Work out the finished part from the listing and answer in its coordinate system (mm). A direction names the side the tool comes from. Coordinates: 2 decimals unless noted, no trailing zeros. Loops run counter-clockwise (first coordinate to the right, second up) from the corner with the lowest first, then second, coordinate; pieces in that order, holes last. Notation, with made-up numbers: (85, 66) -> (136, 66) arc R23 ccw to (136, 86) -> close; hole circle Ø1 at (-11, 58). An arc over 180 degrees is marked (long way). Use a Markdown table: item, result.
from build123d import *

# Parameters (mm, degrees)
PAD003_DEPTH    = 975
SKETCH013_W     = 310
SKETCH013_H     = 1100
SKETCH013_W_2   = 5
SKETCH013_H_2   = 42.9
POCKET007_DEPTH = 50
SKETCH014_W     = 24.5
SKETCH014_H     = 38.9
POCKET008_DEPTH = 5
PAD004_DEPTH    = 5


with BuildPart() as part:
    # Sketch012 → Pad003 (new body)
    with BuildSketch(Plane.XZ):
        with BuildLine():
            add(Edge.make_bspline(
                [(300, 0), (299.662763, 0.037038), (298.339429, 0.190429), (295.439956, 0.589667), (290.775356, 1.337839), (284.500044, 2.393262), (276.735212, 3.66473), (267.577355, 5.083019), (257.136483, 6.653879), (245.549215, 8.381993), (232.975291, 10.222771), (219.590016, 12.153256), (205.573823, 14.115503), (191.111579, 16.055183), (176.381713, 17.897983), (161.544489, 19.553409), (146.739309, 20.940939), (132.087536, 21.99009), (117.705275, 22.664279), (103.703346, 22.961168), (90.192549, 22.858072), (77.284675, 22.375726), (65.094168, 21.544938), (53.730431, 20.369385), (43.29002, 18.857963), (33.852484, 17.043697), (25.485501, 14.967735), (18.252292, 12.67281), (12.179436, 10.224412), (7.338355, 7.689021), (3.623023, 5.152403), (1.3546, 2.748114), (-0.314638, 0.590402), (0.575789, -1.804065), (3.482069, -2.72942), (7.386052, -3.91761), (13.030922, -4.754284), (20.096342, -5.463024), (28.645402, -5.933379), (38.56853, -6.201185), (49.790194, -6.284208), (62.196701, -6.193111), (75.660953, -5.967607), (90.034637, -5.629522), (105.153445, -5.226063), (120.83724, -4.775199), (136.895942, -4.296045), (153.13493, -3.818601), (169.356828, -3.345106), (185.36574, -2.889379), (200.968742, -2.465331), (215.974941, -2.074889), (230.201502, -1.715375), (243.47905, -1.394255), (255.639348, -1.103787), (266.558709, -0.84997), (276.034546, -0.603516), (284.209016, -0.340421), (290.324818, -0.117753), (295.956469, 0.021784), (297.365519, 0.017012), (300.344672, 0.018536), (300.000994, -0.000109), (300, 0)],
                knots=[0, 0, 0, 0, 1.017748, 3.99659, 8.779341, 15.189917, 23.087031, 32.383824, 42.990765, 54.76218, 67.530065, 81.114584, 95.333435, 109.988542, 124.889458, 139.866624, 154.774633, 169.496697, 183.930349, 197.964304, 211.506735, 224.45797, 236.709214, 248.156653, 258.723012, 268.346769, 276.97692, 284.567784, 291.102108, 296.573756, 300.992679, 304.39163, 306.761357, 308.43213, 311.131254, 315.298227, 320.951765, 328.080828, 336.654655, 346.609821, 357.866231, 370.316475, 383.83025, 398.264023, 413.449345, 429.202773, 445.334827, 461.646891, 477.940787, 494.021253, 509.693044, 524.767168, 539.054704, 552.387642, 564.607107, 575.560217, 585.109622, 593.180747, 599.700326, 604.53767, 607.540683, 608.560842, 608.563842, 608.563842, 608.563842, 608.563842], degree=3))
        make_face()
    extrude(amount=PAD003_DEPTH)

    # Sketch013 → Pocket007 (cut, symmetric)
    with BuildSketch(Plane.XY):
        with Locations((155, -550)):
            Rectangle(SKETCH013_W, SKETCH013_H)
        with Locations((104.55, -28.45)):
            Rectangle(SKETCH013_W_2, SKETCH013_H_2, mode=Mode.SUBTRACT)
    extrude(amount=POCKET007_DEPTH, both=True, mode=Mode.SUBTRACT)

    # Sketch014 (on Face3 of Pocket007) → Pocket008 (cut)
    with BuildSketch(Plane(origin=(107.05, 0, 0), x_dir=(0, 0, 1), z_dir=(1, 0, 0))):
        with Locations((8.777474, 28.45)):
            Rectangle(SKETCH014_W, SKETCH014_H)
    extrude(amount=-POCKET008_DEPTH, mode=Mode.SUBTRACT)

    # Sketch015 (on Face3 of Pocket008) → Pad004 (join)
    with BuildSketch(Plane(origin=(107.05, 0, 0), x_dir=(0, 0, 1), z_dir=(1, 0, 0))):
        Polygon((-4.239797, 34.207994), (22.004584, 23.751485), (22.004584, 21.598585), (-4.239797, 32.055093), align=None)
    extrude(amount=-PAD004_DEPTH)


solid = part.part
Q1. For faces 3 (the flat face through (105, -41, -3.473)), 4 (the flat face through (105, -49.9, 9)), determine the directions among +Z, -Z, +X, -X, +Y, -Y from which every point of the face is accessible in a straight line to the end or side of a thin tool.
Solved:
| item | result |
|---|---|
| face 3 | +X, -X |
| face 4 | +Z, -Z, +X, -X, -Y |
Q2. Section A-A on z = 17.75 is taken. Determine the outline of the cut face in (x, y), and give its area (3 significant figures).
Solved:
| item | result |
|---|---|
| outline | (102.05, -49.9) -> (107.05, -49.9) -> (107.05, -47.9) -> (102.05, -47.9) -> close; (102.05, -25.45) -> (107.05, -25.45) -> (107.05, -23.29) -> (102.05, -23.29) -> close; (102.05, -9) -> (107.05, -9) -> (107.05, -7) -> (102.05, -7) -> close |
| area | 30.8 mm² |
Q3. Section B-B on y = -25.5 is taken. State how many separate pieces and enclosed holes the cut face has, and give its area (3 significant figures).
Solved:
| item | result |
|---|---|
| separate pieces | 3 |
| enclosed holes | 0 |
| area | 45.1 mm² |
Q4. Given pin 1 Ø1.5 at (x, y) = (104, -31.5) entering from -Z, flat-ended and moving along its own axis, determine where the tip first touches the part or whether it passes through.
Solved:
| item | result |
|---|---|
| pin 1 | z = -5.27 |
Q5. Determine the mould class of faces 1 (the flat face through (104.58, -26.8, 8.95)), 2 (the flat face through (102.05, -27, 10)) for opening direction Z: pulls with the +Z half, pulls with the -Z half, needs draft (parallel to the pull), parting line crosses it, or undercut.
Solved:
| item | result |
|---|---|
| face 1 | undercut |
| face 2 | needs draft |
Q6. Consider line 1 (Z direction, x = 106.7, y = -21.5); line 2 (Y direction, x = 105.65, z = 19.5); line 3 (Y direction, x = 106, z = 20.5). Determine where each line is inside the solid, lowest interval first. Write a range as [from, to].
Solved:
| item | result |
|---|---|
| line 1 | [-5.18, -3.47], [21.03, 22.87] |
| line 2 | [-49.9, -47.9], [-24.75, -22.6], [-9, -7] |
| line 3 | [-49.9, -47.9], [-24.35, -22.2], [-9, -7] |
